Geometry: final body of the model. Coordinates: model frame, mm. A direction names the side the tool comes from. Give positions to 0.01 mm unless a question says otherwise; leave off trailing zeros. Loops run counter-clockwise (first coordinate to the right, second up) from the corner with the lowest first, then second, coordinate; pieces in that order, holes last. Notation, with made-up numbers: M 30.25,62.5 L 66.25,62.5 A36 cw 66.25,100.5 Z; hole C -26.5,16.5 d6. An arc over 180 degrees is marked long. Put each result on its own line as item: value.
```python
from build123d import *

# Parameters (mm, degrees)
SKETCH1_R            = 10
BOSS_EXTRUDE1_DEPTH  = 3
SKETCH2_R            = 5
BOSS_EXTRUDE2_DEPTH  = 100
CUT_EXTRUDE1_DEPTH   = 15
SKETCH4_W            = 14
SKETCH4_H            = 100
BOSS_EXTRUDE3_DEPTH  = 90
BOSS_EXTRUDE4_START  = 5
SKETCH5_R            = 10
BOSS_EXTRUDE4_DEPTH  = 3
SKETCH7_W            = 31.538450714
SKETCH7_H            = 13
CUT_EXTRUDE2_DEPTH   = 80
SKETCH8_W            = 9
SKETCH8_H            = 87
CUT_EXTRUDE3_DEPTH   = 130
SKETCH9_W            = 9
SKETCH9_H            = 25
CUT_EXTRUDE4_DEPTH   = 80
SKETCH10_W           = 37.5
SKETCH10_H           = 3
BOSS_EXTRUDE5_DEPTH  = 6
SKETCH11_R           = 1.1
CUT_EXTRUDE5_DEPTH   = 56
SKETCH14_W           = 15
SKETCH14_H           = 19.5
CUT_EXTRUDE6_DEPTH   = 56
FILLET1_R            = 3
SKETCH19_W           = 5
SKETCH19_H           = 100
BOSS_EXTRUDE6_DEPTH  = 25
SKETCH22_W           = 5
SKETCH22_H           = 115
BOSS_EXTRUDE8_DEPTH  = 20
SKETCH23_W           = 5
SKETCH23_H           = 115
BOSS_EXTRUDE9_DEPTH  = 20
SKETCH24_W           = 140
SKETCH24_H           = 95
BOSS_EXTRUDE10_DEPTH = 15
SKETCH25_W           = 130
SKETCH25_H           = 90
CUT_EXTRUDE7_DEPTH   = 10
FILLET2_R            = 3
SKETCH26_W           = 2.5
SKETCH26_H           = 95
CUT_EXTRUDE8_DEPTH   = 130
SKETCH27_W           = 2.5
SKETCH27_H           = 10
CUT_EXTRUDE9_DEPTH   = 136.255314129


with BuildPart() as part:
    # Sketch1 → Boss-Extrude1 (new body)
    with BuildSketch(Plane(origin=(0, 0, 0), x_dir=(1, 0, 0), z_dir=(0, 1, 0))):
        with Locations(Location((0, 0, 0), (0, 0, 270))):
            Circle(SKETCH1_R)
    extrude(amount=BOSS_EXTRUDE1_DEPTH)

    # Sketch2 → Boss-Extrude2 (add)
    with BuildSketch(Plane(origin=(0, 3, 0), x_dir=(1, 0, 0), z_dir=(0, 1, 0))):
        with Locations(Location((0, 0, 0), (0, 0, 270))):
            Circle(SKETCH2_R)
    extrude(amount=BOSS_EXTRUDE2_DEPTH)

    # Sketch3 → Cut-Extrude1 (cut)
    with BuildSketch(Plane.XZ):
        with BuildLine():
            ThreePointArc((-1.889982989, -1.636448686), (2.5, 0), (-1.889982989, 1.636448686))
            Line((-1.889982989, 1.636448686), (-1.889982989, -1.636448686))
        make_face()
    extrude(amount=-CUT_EXTRUDE1_DEPTH, mode=Mode.SUBTRACT)

    # Sketch4 → Boss-Extrude3 (add)
    with BuildSketch(Plane(origin=(0, 103, 0), x_dir=(1, 0, 0), z_dir=(0, 1, 0))):
        Rectangle(SKETCH4_W, SKETCH4_H)
    extrude(amount=-BOSS_EXTRUDE3_DEPTH)

    # Sketch5 → Boss-Extrude4 (add)
    with BuildSketch(Plane(origin=(0, 3, 0), x_dir=(1, 0, 0), z_dir=(0, 1, 0)).offset(BOSS_EXTRUDE4_START)):
        with Locations(Location((0, 0, 0), (0, 0, 270))):
            Circle(SKETCH5_R)
    extrude(amount=BOSS_EXTRUDE4_DEPTH)

    # Sketch7 → Cut-Extrude2 (cut)
    with BuildSketch(Plane.XY.offset(50)):
        with Locations((1.592851046, 6.5)):
            Rectangle(SKETCH7_W, SKETCH7_H)
    extrude(amount=-CUT_EXTRUDE2_DEPTH, mode=Mode.SUBTRACT)

    # Sketch8 → Cut-Extrude3 (cut)
    with BuildSketch(Plane.XY.offset(50)):
        with Locations((2.5, 59.5)):
            Rectangle(SKETCH8_W, SKETCH8_H)
    extrude(amount=-CUT_EXTRUDE3_DEPTH, mode=Mode.SUBTRACT)

    # Sketch9 → Cut-Extrude4 (cut)
    with BuildSketch(Plane(origin=(0, 16, 0), x_dir=(1, 0, 0), z_dir=(0, 1, 0))):
        with Locations((2.5, 0)):
            Rectangle(SKETCH9_W, SKETCH9_H)
    extrude(amount=-CUT_EXTRUDE4_DEPTH, mode=Mode.SUBTRACT)

    # Sketch10 → Boss-Extrude5 (add)
    with BuildSketch(Plane(origin=(7, 0, 0), x_dir=(0, 0, -1), z_dir=(1, 0, 0))):
        with Locations((-31.25, 14.5)):
            Rectangle(SKETCH10_W, SKETCH10_H)
        with Locations((31.25, 14.5)):
            Rectangle(SKETCH10_W, SKETCH10_H)
    extrude(amount=BOSS_EXTRUDE5_DEPTH)

    # Sketch11 → Cut-Extrude5 (cut)
    with BuildSketch(Plane(origin=(0, 16, 0), x_dir=(1, 0, 0), z_dir=(0, 1, 0))):
        with Locations(Location((5.5, -17, 0), (0, 0, 270))):
            Circle(SKETCH11_R)
        with Locations(Location((5.5, -20, 0), (0, 0, 270))):
            Circle(SKETCH11_R)
        with Locations(Location((5.5, -23, 0), (0, 0, 270))):
            Circle(SKETCH11_R)
        with Locations(Location((5.5, -26, 0), (0, 0, 270))):
            Circle(SKETCH11_R)
        with Locations(Location((5.5, 26, 0), (0, 0, 270))):
            Circle(SKETCH11_R)
        with Locations(Location((5.5, 23, 0), (0, 0, 270))):
            Circle(SKETCH11_R)
        with Locations(Location((5.5, 20, 0), (0, 0, 270))):
            Circle(SKETCH11_R)
        with Locations(Location((5.5, 17, 0), (0, 0, 270))):
            Circle(SKETCH11_R)
    extrude(amount=-CUT_EXTRUDE5_DEPTH, mode=Mode.SUBTRACT)

    # Sketch14 → Cut-Extrude6 (cut)
    with BuildSketch(Plane(origin=(0, 16, 0), x_dir=(1, 0, 0), z_dir=(0, 1, 0))):
        with Locations((5.5, -40.25)):
            Rectangle(SKETCH14_W, SKETCH14_H)
        with Locations((5.5, 40.25)):
            Rectangle(SKETCH14_W, SKETCH14_H)
    extrude(amount=-CUT_EXTRUDE6_DEPTH, mode=Mode.SUBTRACT)

    # Fillet1
    fillet1_edges = [part.edges().sort_by_distance(p)[0] for p in [
        (-2, 16, 21.5),
        (-2, 14.5, 12.5),
        (-2, 14.5, -12.5),
        (13, 14.5, 12.5),
        (13, 14.5, -12.5),
        (13, 14.5, -30.5),
        (13, 14.5, 30.5),
        (-2, 16, -21.5),
        (-2, 14.5, 30.5),
        (-2, 14.5, -30.5),
    ]]
    fillet(fillet1_edges, radius=FILLET1_R)

    # Sketch19 → Boss-Extrude6 (add)
    with BuildSketch(Plane(origin=(0, 103, 0), x_dir=(1, 0, 0), z_dir=(0, 1, 0))):
        with Locations((-4.5, 0)):
            Rectangle(SKETCH19_W, SKETCH19_H)
    extrude(amount=BOSS_EXTRUDE6_DEPTH)

    # Sketch22 → Boss-Extrude8 (add)
    with BuildSketch(Plane.XY.offset(50)):
        with Locations((-4.5, 70.5)):
            Rectangle(SKETCH22_W, SKETCH22_H)
    extrude(amount=BOSS_EXTRUDE8_DEPTH)

    # Sketch23 → Boss-Extrude9 (add)
    with BuildSketch(Plane(origin=(0, 0, -50), x_dir=(-1, 0, 0), z_dir=(0, 0, -1))):
        with Locations((4.5, 70.5)):
            Rectangle(SKETCH23_W, SKETCH23_H)
    extrude(amount=BOSS_EXTRUDE9_DEPTH)

    # Sketch24 → Boss-Extrude10 (add)
    with BuildSketch(Plane(origin=(-2, 0, 0), x_dir=(0, 0, -1), z_dir=(1, 0, 0))):
        with Locations((0, 80.5)):
            Rectangle(SKETCH24_W, SKETCH24_H)
    extrude(amount=BOSS_EXTRUDE10_DEPTH)

    # Sketch25 → Cut-Extrude7 (cut)
    with BuildSketch(Plane.ZY.offset(7)):
        with Locations((0, 80.5)):
            Rectangle(SKETCH25_W, SKETCH25_H)
    extrude(amount=-CUT_EXTRUDE7_DEPTH, mode=Mode.SUBTRACT)

    # Fillet2
    fillet2_edges = [part.edges().sort_by_distance(p)[0] for p in [
        (-2, 33, 0),
    ]]
    fillet(fillet2_edges, radius=FILLET2_R)

    # Sketch26 → Cut-Extrude8 (cut)
    with BuildSketch(Plane.XY.offset(70)):
        with Locations((11.75, 80.5)):
            Rectangle(SKETCH26_W, SKETCH26_H)
    extrude(amount=-CUT_EXTRUDE8_DEPTH, mode=Mode.SUBTRACT)

    # Sketch27 → Cut-Extrude9 (cut, through all)
    with BuildSketch(Plane(origin=(0, 128, 0), x_dir=(1, 0, 0), z_dir=(0, 1, 0))):
        with Locations((11.75, 65)):
            Rectangle(SKETCH27_W, SKETCH27_H)
    extrude(amount=-CUT_EXTRUDE9_DEPTH, mode=Mode.SUBTRACT)


solid = part.part
```
Item 1: Pin query (flat end, axial travel): pin 1 Ø4 at (x, z) = (3.5, -50.5) entering from -Y; pin 2 Ø1.5 at (y, z) = (112.5, 39.5) entering from -X; pin 3 Ø12 at (y, z) = (90.5, 40) entering from +X; pin 4 Ø2.5 at (x, z) = (5.5, -26) entering from -Y. Return the tip coordinate at first contact, or that it passes through.
Output values:
pin 1: y = 33
pin 2: x = 3
pin 3: x = 10.5
pin 4: y = 13
Item 2: Set-up query: faces 1 (the flat face through (10.5, 80, 1)), 2 (the flat face through (-2, 35.5, -1)), 3 (the flat face through (5, 15, -12.5)). Return all of +Z, -Z, +X, -X, +Y, -Y with unobstructed straight access to the full face (end or side cutting, diameter ignored); none if empty.
Output values:
face 1: +Z, -Z, +X, +Y
face 2: -X
face 3: +X, -Y
Item 3: Section D-D on y = 31.5. Output: boundary loops of the cut face in (x, z).
Output values:
outline: M -7,-70 L -1.6,-70 L -1.6,70 L -7,70 Z
Item 4: Section B-B on y = 85.5. Output: boundary loops of the cut face in (x, z), then the cut area to 3 significant figures.
Output values:
outline: M -7,-70 L 10.5,-70 L 10.5,70 L -7,70 L -7,65 L 3,65 L 3,-65 L -7,-65 Z
area: 1,150 mm²
Item 5: Section A-A on x = -4.5. Output: boundary loops of the cut face in (y, z).
Output values:
outline: M 13,-70 L 128,-70 L 128,70 L 13,70 Z; hole M 35.5,-65 L 125.5,-65 L 125.5,65 L 35.5,65 Z
Item 6: Mould query, pull axis Z, two halves, no side actions, for faces 4 (the flat face through (7, 16, -21)), 5 (the cylindrical face through (-1.48, 15.29, 31.81)), 6 (the cylindrical face through (12.14, 14.52, -13.4)), 7 (the flat face through (-2, 125.5, -1)). Classes: pulls with the +Z half, pulls with the -Z half, needs draft (parallel to the pull), parting line crosses it, or undercut.
Output values:
face 4: needs draft
face 5: pulls with the +Z half
face 6: undercut
face 7: undercut
Item 7: Line query: probe 1 along Y at (x, z) = (2.75, -17); probe 2 along Z at (x, y) = (-0.5, 78); probe 3 along Y at (x, z) = (-5.25, -56.5). Output: solid intervals per line, ascending. Write a range as [from, to].
Output values:
probe 1: [13, 16], [33, 35.5], [125.5, 128]
probe 2: [-70, -65], [65, 70]
probe 3: [13, 35.5], [125.5, 128]
Item 8: Section C-C on z = -53.5. Output: boundary loops of the cut face in (x, y), then the cut area to 3 significant figures.
Output values:
outline: M -7,13 L -2,13 L -2,30 A3 cw 1,33 L 10.5,33 L 10.5,128 L -7,128 L -7,125.5 L 3,125.5 L 3,35.5 L -7,35.5 Z
area: 864 mm²
